from build123d import *

# Parameters (mm, degrees)
SKETCH_1_R           = 3
SKETCH_1_W           = 90
SKETCH_1_H           = 120
SKETCH_1_R_2         = 10
SKETCH_1_R_3         = 7.5
EXTRUDE_2_DEPTH      = 3
EXTRUDE_START        = -10
SKETCH_2_R           = 7.5
EXTRUDE_3_DEPTH      = 10
CUT_EXTRUDE_1_DEPTH  = 10
EXTRUDE_START_2      = -3
SKETCH_4_R           = 10
EXTRUDE_4_DEPTH      = 3
SKETCH_6_W           = 7
SKETCH_6_H           = 14.142135624
CUT_EXTRUDE_5_DEPTH  = 333.489097566
SKETCH_7_W           = 90
SKETCH_7_H           = 120
EXTRUDE_5_DEPTH      = 3
SKETCH_8_W           = 10
SKETCH_8_H           = 50
EXTRUDE_6_DEPTH      = 30
SKETCH_9_R           = 8
CUT_EXTRUDE_6_DEPTH  = 30
SKETCH_10_R          = 3
EXTRUDE_7_DEPTH      = 3
SKETCH_11_R          = 3
CUT_EXTRUDE_7_DEPTH  = 3
SKETCH_12_R          = 3
EXTRUDE_8_DEPTH      = 3
SKETCH_13_R          = 3
CUT_EXTRUDE_8_DEPTH  = 3
SKETCH_14_R          = 3
CUT_EXTRUDE_9_DEPTH  = 10
SKETCH_15_R          = 3
CUT_EXTRUDE_10_DEPTH = 231.922064775
SKETCH_16_R          = 3
EXTRUDE_10_DEPTH     = 3
SKETCH_17_R          = 3
CUT_EXTRUDE_11_DEPTH = 231.922064775
SKETCH_18_R          = 5
CUT_EXTRUDE_12_DEPTH = 10
SKETCH_20_R          = 1.5
CUT_EXTRUDE_13_DEPTH = 10
CUT_EXTRUDE_14_DEPTH = 10


with BuildPart() as part:
    # 草图1 → 凸台-拉伸2 (new body)
    # profile 1 of 9: a face of its own
    with BuildSketch(Plane.XY):
        Polygon((195, -115), (195, 115), (190, 115), (190, 120), (115, 120), (115, 75), (75, 75), (-90, 75), (-130, 75), (-130, 120), (-175, 120), (-175, 90), (-195, 90), (-195, -90), (-175, -90), (-175, -120), (-130, -120), (-130, -75), (-90, -75), (75, -75), (115, -75), (115, -120), (190, -120), (190, -115), align=None)
        with Locations((-184.089468205, -70)):
            Circle(SKETCH_1_R, mode=Mode.SUBTRACT)
        with Locations((-87, -69)):
            Circle(SKETCH_1_R, mode=Mode.SUBTRACT)
        with Locations((-184.089468205, 70)):
            Circle(SKETCH_1_R, mode=Mode.SUBTRACT)
        with Locations((-87, 69)):
            Circle(SKETCH_1_R, mode=Mode.SUBTRACT)
        Rectangle(SKETCH_1_W, SKETCH_1_H, mode=Mode.SUBTRACT)
        with Locations((75, 0)):
            Circle(SKETCH_1_R_2, mode=Mode.SUBTRACT)
        with Locations((117.5, 0)):
            Circle(SKETCH_1_R_3, mode=Mode.SUBTRACT)
    # profile 2 of 9: a face of its own
    with BuildSketch(Plane.XY):
        Polygon((-130, 120), (-90, 75), (-130, 75), align=None)
    # profile 3 of 9: a face of its own
    with BuildSketch(Plane.XY):
        Polygon((-175, 120), (-175, 90), (-195, 90), align=None)
    # profile 4 of 9: a face of its own
    with BuildSketch(Plane.XY):
        Polygon((-175, -120), (-195, -90), (-175, -90), align=None)
    # profile 5 of 9: a face of its own
    with BuildSketch(Plane.XY):
        Polygon((-130, -120), (-130, -75), (-90, -75), align=None)
    # profile 6 of 9: a face of its own
    with BuildSketch(Plane.XY):
        Polygon((115, -120), (75, -75), (115, -75), align=None)
        with Locations((104.379549532, -93)):
            Circle(SKETCH_1_R, mode=Mode.SUBTRACT)
    # profile 7 of 9: a face of its own
    with BuildSketch(Plane.XY):
        Polygon((115, 120), (115, 75), (75, 75), align=None)
        with Locations((104.379549532, 93)):
            Circle(SKETCH_1_R, mode=Mode.SUBTRACT)
    # profile 8 of 9: a face of its own
    with BuildSketch(Plane.XY):
        Polygon((190, 120), (195, 115), (190, 115), align=None)
    # profile 9 of 9: a face of its own
    with BuildSketch(Plane.XY):
        Polygon((190, -115), (190, -120), (195, -115), align=None)
    extrude(amount=EXTRUDE_2_DEPTH)

    # 草图2 → 凸台-拉伸3 (add)
    with BuildSketch(Plane.XY.offset(3).offset(EXTRUDE_START)):
        with Locations((117.5, 0)):
            Circle(SKETCH_2_R)
    extrude(amount=EXTRUDE_3_DEPTH)

    # 草图3 → 切除-拉伸1 (cut)
    with BuildSketch(Plane.XY.offset(3)):
        Polygon((115, 120), (115, -120), (190, -120), (195, -115), (195, 115), (190, 120), align=None)
        Polygon((115, -120), (115, -114.375), (110, -114.375), align=None)
        Polygon((115, 114.376866735), (115, 120), (110.00165932, 114.376866735), align=None)
    extrude(amount=-CUT_EXTRUDE_1_DEPTH, mode=Mode.SUBTRACT)

    # 草图4 → 凸台-拉伸4 (add)
    with BuildSketch(Plane.XY.offset(3).offset(EXTRUDE_START_2)):
        with Locations((75, 0)):
            Circle(SKETCH_4_R)
    extrude(amount=EXTRUDE_4_DEPTH)

    # 草图6 → 切除-拉伸5 (cut, through all)
    with BuildSketch(Plane(origin=(115, 0, 0), x_dir=(0, 0, -1), z_dir=(1, 0, 0))):
        with Locations((3.5, 0)):
            Rectangle(SKETCH_6_W, SKETCH_6_H)
    extrude(amount=-CUT_EXTRUDE_5_DEPTH, mode=Mode.SUBTRACT)

    # 草图7 → 凸台-拉伸5 (add)
    with BuildSketch(Plane.XY.offset(3)):
        Rectangle(SKETCH_7_W, SKETCH_7_H)
    extrude(amount=-EXTRUDE_5_DEPTH)

    # 草图8 → 凸台-拉伸6 (add)
    with BuildSketch(Plane.XY.offset(3)):
        with Locations((110, 0)):
            Rectangle(SKETCH_8_W, SKETCH_8_H)
    extrude(amount=EXTRUDE_6_DEPTH)

    # 草图9 → 切除-拉伸6 (cut)
    with BuildSketch(Plane(origin=(115, 0, 0), x_dir=(0, 0, -1), z_dir=(1, 0, 0))):
        with Locations((-17.93158575, 0)):
            Circle(SKETCH_9_R)
    extrude(amount=-CUT_EXTRUDE_6_DEPTH, mode=Mode.SUBTRACT)

    # 草图10 → 凸台-拉伸7 (add)
    with BuildSketch(Plane.XY.offset(3).offset(EXTRUDE_START_2)):
        with Locations((104.379549532, -93)):
            Circle(SKETCH_10_R)
        with Locations((104.379549532, 93)):
            Circle(SKETCH_10_R)
    extrude(amount=EXTRUDE_7_DEPTH)

    # 草图11 → 切除-拉伸7 (cut)
    with BuildSketch(Plane.XY.offset(3)):
        with Locations((100, -88.073006777)):
            Circle(SKETCH_11_R)
        with Locations(Location((100, 88.073006777, 0), (0, 0, 180))):
            Circle(SKETCH_11_R)
    extrude(amount=-CUT_EXTRUDE_7_DEPTH, mode=Mode.SUBTRACT)

    # 草图12 → 凸台-拉伸8 (add)
    with BuildSketch(Plane.XY.offset(3).offset(EXTRUDE_START_2)):
        with Locations((-87, 69)):
            Circle(SKETCH_12_R)
        with Locations((-87, -69)):
            Circle(SKETCH_12_R)
    extrude(amount=EXTRUDE_8_DEPTH)

    # 草图13 → 切除-拉伸8 (cut)
    with BuildSketch(Plane.XY.offset(3)):
        with Locations((-90, 65)):
            Circle(SKETCH_13_R)
        with Locations(Location((-90, -65, 0), (0, 0, 180))):
            Circle(SKETCH_13_R)
    extrude(amount=-CUT_EXTRUDE_8_DEPTH, mode=Mode.SUBTRACT)

    # 草图14 → 切除-拉伸9 (cut)
    with BuildSketch(Plane.XY.offset(3)):
        with BuildLine():
            ThreePointArc((-159.5, 88), (-160.378679656, 90.121320344), (-162.5, 91))
            Line((-162.5, 91), (-162.5, 85))
            ThreePointArc((-162.5, 85), (-160.378679656, 85.878679656), (-159.5, 88))
        make_face()
        with BuildLine():
            Line((-162.5, 85), (-162.5, 91))
            ThreePointArc((-162.5, 91), (-165.5, 88), (-162.5, 85))
        make_face()
        with Locations((-162.5, -88)):
            Circle(SKETCH_14_R)
    extrude(amount=-CUT_EXTRUDE_9_DEPTH, mode=Mode.SUBTRACT)

    # 草图15 → 切除-拉伸10 (cut, through all)
    with BuildSketch(Plane.XY.offset(3)):
        with Locations((-162.5, -93)):
            Circle(SKETCH_15_R)
        with Locations((-162.5, -88)):
            Circle(SKETCH_15_R)
        with Locations((-162.5, 93)):
            Circle(SKETCH_15_R)
        with Locations((-162.5, 88)):
            Circle(SKETCH_15_R)
    extrude(amount=-CUT_EXTRUDE_10_DEPTH, mode=Mode.SUBTRACT)

    # 草图16 → 凸台-拉伸10 (add)
    with BuildSketch(Plane.XY.offset(3)):
        with Locations((-162.5, 88)):
            Circle(SKETCH_16_R)
        with Locations((-162.5, -88)):
            Circle(SKETCH_16_R)
    extrude(amount=-EXTRUDE_10_DEPTH)

    # 草图17 → 切除-拉伸11 (cut, through all)
    with BuildSketch(Plane.XY.offset(3)):
        with Locations((-162.5, 93)):
            Circle(SKETCH_17_R)
        with Locations((-162.5, -93)):
            Circle(SKETCH_17_R)
    extrude(amount=-CUT_EXTRUDE_11_DEPTH, mode=Mode.SUBTRACT)

    # 草图18 → 切除-拉伸12 (cut)
    with BuildSketch(Plane.XY.offset(3)):
        with Locations((-170, 22.5)):
            Circle(SKETCH_18_R)
        with Locations((-170, -22.5)):
            Circle(SKETCH_18_R)
    extrude(amount=-CUT_EXTRUDE_12_DEPTH, mode=Mode.SUBTRACT)

    # 草图20 → 切除-拉伸13 (cut)
    with BuildSketch(Plane.XY.offset(3)):
        Circle(SKETCH_20_R)
    extrude(amount=-CUT_EXTRUDE_13_DEPTH, mode=Mode.SUBTRACT)

    # 草图21 → 切除-拉伸14 (cut)
    with BuildSketch(Plane.XY.offset(3)):
        with BuildLine():
            ThreePointArc((-182.25, 0), (-183.421572875, 2.828427125), (-186.25, 4))
            Line((-186.25, 4), (-186.25, -4))
            ThreePointArc((-186.25, -4), (-183.421572875, -2.828427125), (-182.25, 0))
        make_face()
        with BuildLine():
            Line((-186.25, -4), (-186.25, 4))
            ThreePointArc((-186.25, 4), (-190.25, 0), (-186.25, -4))
        make_face()
    extrude(amount=-CUT_EXTRUDE_14_DEPTH, mode=Mode.SUBTRACT)


solid = part.part
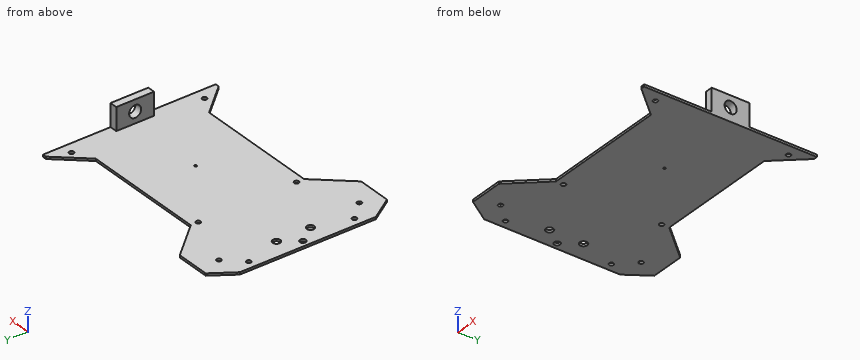
The listing builds one solid part. Answer for the finished solid, in the listing's coordinates (mm). Round coordinates to 2 decimals unless told otherwise and drop trailing zeros. Loops run counter-clockwise (first coordinate to the right, second up) from the corner with the lowest first, then second, coordinate; pieces in that order, holes last. Notation, with made-up numbers: M -8.5,-18.5 L 46.5,-18.5 A24 cw 46.5,17.5 Z; hole C 31.25,62 d9. An arc over 180 degrees is marked long. Write each question's results on one line, items separated by ' | '. Start each with the question number.
1) Find section A-A on x = -170. Write down the section's boundary in (y, z).
2) Straight lines are drawn through the part: probe 1 along Y at (x, z) = (-170, 1.8); probe 2 along Z at (x, y) = (0, -25.5); probe 3 along X at (y, z) = (-19.5, 25.5). For each, find the intervals that lie inside material, in ascending order.
3) Find section B-B on z = 21.5. Write down the section's boundary in (x, y).
4) Each of these flat-tipped pins is pushed along its axis until it touches: pin 1 (8 mm diameter, centred on x = -170, y = 22.5, fed in from +Z); pin 2 (0.9 mm diameter, centred on x = 112.5, z = 2, fed in from +Y); pin 3 (3 mm diameter, centred on x = 112, z = 12, fed in from -Y); pin 4 (9.5 mm diameter, centred on x = -90, y = -65, fed in from +Z). Where does it stop, or does it pass through?
5) Find section D-D on y = 49. Write down the section's boundary in (x, z), plus the area to 3 significant figures.
6) Find section C-C on y = 81. Write down the section's boundary in (x, z).
Final values:
1) outline: M -120,0 L -27.5,0 L -27.5,3 L -120,3 Z; M -17.5,0 L 17.5,0 L 17.5,3 L -17.5,3 Z; M 27.5,0 L 120,0 L 120,3 L 27.5,3 Z
2) probe 1: -120 to -27.5, -17.5 to 17.5, 27.5 to 120 | probe 2: 0 to 3 | probe 3: 105 to 115
3) outline: M 105,-25 L 115,-25 L 115,-7.16 L 105,-7.16 Z; M 105,7.16 L 115,7.16 L 115,25 L 105,25 Z
4) pin 1: through | pin 2: y = 114.38 | pin 3: y = -25 | pin 4: z = 3
5) outline: M -195,0 L 115,0 L 115,3 L -195,3 Z | area: 930 mm²
6) outline: M -195,0 L -95.33,0 L -95.33,3 L -195,3 Z; M 80.33,0 L 115,0 L 115,3 L 80.33,3 Z
